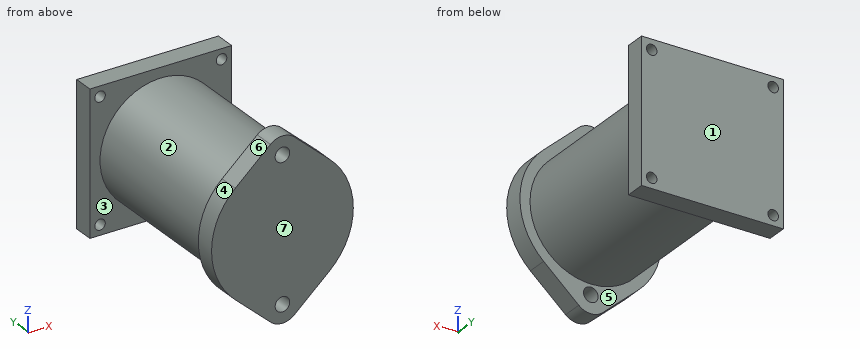
Autodesk Inventor part; units mm, degrees
ref_plane "YZ Plane" through (0, 0, 0) normal (1, 0, 0) x (0, 1, 0)
ref_plane "XZ Plane" through (0, 0, 0) normal (0, 1, 0) x (-1, 0, 0)
ref_plane "XY Plane" through (0, 0, 0) normal (0, 0, 1) x (1, 0, 0)
sketch "Boceto1" plane through (0, 0, 0) normal (0, 1, 0) x (-1, 0, 0)
  circle A0 centre (0, 0) radius 32.5
  arc A1 (23.3059, -26.112) -> (23.3059, 26.112) centre (0, 0) ccw
  circle A2 centre (0, -35) radius 3.6
  circle A3 centre (0, 0) radius 43.5
  arc A4 (8.153, -31.4608) -> (-5.9184, -41.631) centre (0, -35) ccw
  line L0 (23.3059, -26.112) -> (5.9184, -41.631)
  line L1 (-23.3059, -26.112) -> (-5.9184, -41.631)
  arc A5 (5.9184, -41.631) -> (8.153, -31.4608) centre (0, -35) ccw
  arc A6 (-5.9184, -41.631) -> (5.9184, -41.631) centre (0, -35) ccw
  line L2 (0, 0) -> (19.418, 0)
  circle A7 centre (0, 35) radius 3.6
  arc A8 (-5.9184, 41.631) -> (8.153, 31.4608) centre (0, 35) ccw
  line L3 (23.3059, 26.112) -> (5.9184, 41.631)
  line L4 (-23.3059, 26.112) -> (-5.9184, 41.631)
  arc A9 (8.153, 31.4608) -> (5.9184, 41.631) centre (0, 35) ccw
  arc A10 (5.9184, 41.631) -> (-5.9184, 41.631) centre (0, 35) ccw
  arc A11 (23.3059, 26.112) -> (-23.3059, 26.112) centre (0, 0) ccw
  arc A12 (-23.3059, 26.112) -> (-23.3059, -26.112) centre (0, 0) ccw
  dimension "d0" = 65
  dimension "d2" = 7.2
  dimension "d3" = 87
extrude "Extrusión1" add sketch "Boceto1" along normal blind 10 contours A0 A4 A8 | A0 A9 A11 A1 L0 A5 | A8 A0 A7 | A0 A7 A11 A9 | A5 A6 A3 A4 A0 A2 | A0 A2 A4 | A8 A11 A7 A0 | A0 A4 L1 A12 A11 A8 | A11 A7 A8 A10 A3 A9 | A9 L3 A11 | A11 L4 A8 | A6 A3 | A3 A10
sketch "Boceto2" plane through (0, 10, 0) normal (0, 1, 0) x (1, 0, 0)
  circle A0 centre (0, 0) radius 30
  dimension "d7" = 60
extrude "Extrusión2" add sketch "Boceto2" along normal blind 82
sketch "Boceto4" plane through (0, 92, 0) normal (0, 1, 0) x (1, 0, 0)
  line L0 (-35, -35) -> (35, -35)
  line L1 (35, -35) -> (35, 35)
  line L2 (35, 35) -> (-35, 35)
  line L3 (-35, 35) -> (-35, -35)
  line L4 (-35, -35) -> (35, 35) construction
  line L5 (35, -35) -> (-35, 35) construction
  line L6 (30, 30) -> (-30, 30)
  line L7 (-30, 30) -> (-30, -30)
  line L8 (-30, -30) -> (30, -30)
  line L9 (30, -30) -> (30, 30)
  line L10 (30, 30) -> (-30, -30) construction
  line L11 (-30, 30) -> (30, -30) construction
  circle A0 centre (-30, 30) radius 2.6
  circle A1 centre (30, 30) radius 2.6
  circle A2 centre (30, -30) radius 2.6
  circle A3 centre (-30, -30) radius 2.6
  point P0 (0, 0)
  dimension "d13" = 70
  dimension "d14" = 70
  dimension "d15" = 60
  dimension "d16" = 5.2
  dimension "d17" = 5.2
  dimension "d18" = 5.2
  dimension "d19" = 5.2
extrude "Extrusión3" add sketch "Boceto4" along normal blind 10 contours L3 L2 L1 L0 | L6 A1 L9 A2 L8 A3 L7 A0
properties part number "ball-fastening"
CAD build for the part. Positions are in the model's coordinates, mm. Face numbers are marked on the shaded views. A direction names the side the tool comes from. Round coordinates to 2 decimals unless told otherwise and drop trailing zeros. Order: outer loops, then holes, each group sorted by start corner. A loop starts at its lowest first (then second) coordinate and runs counter-clockwise, first axis right, second up. Notation, with made-up numbers: (66, 37.25) - (121, 37.25) arc R15 cw to (121, 66.25) - close; hole circle Ø5 at (24, 60). An arc over 180 degrees is marked (long way). Answer in a Markdown table with one row per item. Add a question column.
(1) Drop flat-ended pins along their axis: pin 1 Ø10 at (y, z) = (55.5, 9.5) entering from +X; pin 2 Ø12 at (y, z) = (14, -20) entering from +X; pin 3 Ø8 at (x, y) = (-23.5, 29) entering from +Z. Give the stop position or say it passes through.
(2) 3-axis set-ups, long thin cutter, end or side, ignore diameter. For the marked faces 5, 6 and 7: which of +Z, -Z, +X, -X, +Y, -Y reach the whole face in a straight line?
(3) Mould opens along Y. For the marked faces 1, 2, 3 and 4 say: +Y half, -Y half, draft (parallel to the pull), parting line (faces both ways), or undercut.
(4) Band-saw the part on A-A on x = 0. List the corners of the cut face in (y, z).
(5) Band-saw the part on B-B on z = 0. List the corners of the cut face in (x, y).
(6) Band-saw the part on C-C on y = 44.5. List the corners of the cut face in (x, z).
(7) Band-saw the part on D-D on x = -22. List the corners of the cut face in (y, z), and give its area (3 significant figures).
(8) Probe L1, parallel to Z at x = 0, y = 4.5; L2, parallel to Z at x = 30, y = 95.5. List the from-to ranges inside material, lowest first. Write a range as [from, to].
Data:
| question | item | result |
|---|---|---|
| 1 | pin 1 | stops at x = 29.66 |
| 1 | pin 2 | stops at x = 31.37 |
| 1 | pin 3 | stops at z = 22.8 |
| 2 | face 5 | none |
| 2 | face 6 | +Z, -X, -Y |
| 2 | face 7 | +Z, -Z, +X, -X, -Y |
| 3 | face 1 | +Y half |
| 3 | face 2 | undercut |
| 3 | face 3 | undercut |
| 3 | face 4 | draft |
| 4 | outline | (0, -43.89) - (10, -43.89) - (10, -38.6) - (0, -38.6) - close; (0, -31.4) - (10, -31.4) - (10, -30) - (92, -30) - (92, -35) - (102, -35) - (102, 35) - (92, 35) - (92, 30) - (10, 30) - (10, 31.4) - (0, 31.4) - close; (0, 38.6) - (10, 38.6) - (10, 43.89) - (0, 43.89) - close |
| 5 | outline | (-35, 0) - (35, 0) - (35, 10) - (30, 10) - (30, 92) - (35, 92) - (35, 102) - (-35, 102) - (-35, 92) - (-30, 92) - (-30, 10) - (-35, 10) - close |
| 6 | outline | circle Ø60 at (0, 0) |
| 7 | outline | (0, -27.28) - (10, -27.28) - (10, -20.4) - (92, -20.4) - (92, -35) - (102, -35) - (102, 35) - (92, 35) - (92, 20.4) - (10, 20.4) - (10, 27.28) - (0, 27.28) - close |
| 7 | area | 4,590 mm^2 |
| 8 | L1 | z = [-43.89, -38.6], [-31.4, 31.4], [38.6, 43.89] |
| 8 | L2 | z = [-35, -32.6], [-27.4, 27.4], [32.6, 35] |
